```python
from build123d import *

# Parameters (mm, degrees)
SKETCH_1_R                   = 27.5
SKETCH_1_R_2                 = 17.5
EXTRUDE_1_DEPTH              = 4
SKETCH_2_R                   = 27.5
SKETCH_2_R_2                 = 18.5
EXTRUDE_2_DEPTH              = 5
EXTRUDE_3_DEPTH              = 9
SKETCH_7_R                   = 18.5
CUT_EXTRUDE_4_DEPTH          = 3
SKETCH_13_R                  = 9.5
CUT_EXTRUDE_9_DEPTH          = 7
SKETCH_14_R                  = 8.5
CUT_EXTRUDE_10_DEPTH         = 3
SKETCH_26_W                  = 65.286774434
SKETCH_26_H                  = 13.225755288
CUT_EXTRUDE_11_DEPTH         = 1111
SKETCH_28_R                  = 9.5
SKETCH_28_R_2                = 8.5
EXTRUDE_4_DEPTH              = 2
HOLE_WIZARD_M3_1_D           = 3.2
HOLE_WIZARD_M3_1_CBORE_D     = 6.5
HOLE_WIZARD_M3_1_CBORE_DEPTH = 3.4
PATTERN_CIRCULAR_1_COUNT     = 6
HOLE_WIZARD_M3_2_D           = 3.2
HOLE_WIZARD_M3_2_CBORE_D     = 6.5
HOLE_WIZARD_M3_2_CBORE_DEPTH = 3.4
PATTERN_CIRCULAR_2_COUNT     = 6


with BuildPart() as part:
    # 스케치1 → 보스-돌출1 (new body)
    with BuildSketch(Plane(origin=(0, 0, 0), x_dir=(1, 0, 0), z_dir=(0, 1, 0))):
        Circle(SKETCH_1_R)
        Circle(SKETCH_1_R_2, mode=Mode.SUBTRACT)
    extrude(amount=EXTRUDE_1_DEPTH)

    # 스케치2 → 보스-돌출2 (add)
    with BuildSketch(Plane(origin=(0, 4, 0), x_dir=(1, 0, 0), z_dir=(0, 1, 0))):
        Circle(SKETCH_2_R)
        Circle(SKETCH_2_R_2, mode=Mode.SUBTRACT)
    extrude(amount=EXTRUDE_2_DEPTH)

    # 스케치3 → 보스-돌출3 (add)
    with BuildSketch(Plane(origin=(0, 9, 0), x_dir=(1, 0, 0), z_dir=(0, 1, 0))):
        with BuildLine():
            Line((4.125, 27.188864908), (62.775, 18.290690938))
            ThreePointArc((62.775, 18.290690938), (78.5, 0), (62.775, -18.290690938))
            Line((62.775, -18.290690938), (4.125, -27.188864908))
            ThreePointArc((4.125, -27.188864908), (27.5, 0), (4.125, 27.188864908))
        make_face()
    extrude(amount=-EXTRUDE_3_DEPTH)

    # 스케치7 → 컷-돌출4 (cut)
    with BuildSketch(Plane(origin=(0, 4, 0), x_dir=(1, 0, 0), z_dir=(0, 1, 0))):
        Circle(SKETCH_7_R)
    extrude(amount=-CUT_EXTRUDE_4_DEPTH, mode=Mode.SUBTRACT)

    # 스케치13 → 컷-돌출9 (cut)
    with BuildSketch(Plane.XZ):
        with Locations((60, 0)):
            Circle(SKETCH_13_R)
    extrude(amount=-CUT_EXTRUDE_9_DEPTH, mode=Mode.SUBTRACT)

    # 스케치14 → 컷-돌출10 (cut, through all)
    with BuildSketch(Plane.XZ.offset(-7)):
        with Locations((60, 0)):
            Circle(SKETCH_14_R)
    extrude(amount=-CUT_EXTRUDE_10_DEPTH, mode=Mode.SUBTRACT)

    # 스케치26 → 컷-돌출11 (cut, symmetric)
    with BuildSketch(Plane(origin=(0, 0, 0), x_dir=(0, 0, -1), z_dir=(1, 0, 0))):
        with Locations((-1.179133759, 11.612877644)):
            Rectangle(SKETCH_26_W, SKETCH_26_H)
    extrude(amount=CUT_EXTRUDE_11_DEPTH, both=True, mode=Mode.SUBTRACT)

    # 스케치28 → 보스-돌출4 (add)
    with BuildSketch(Plane.XZ):
        with Locations((60, 0)):
            Circle(SKETCH_28_R)
        with Locations((60, 0)):
            Circle(SKETCH_28_R_2, mode=Mode.SUBTRACT)
    extrude(amount=-EXTRUDE_4_DEPTH)

    # M3 육각 소켓 머리 캡 나사용 카운터보어1 (through all)
    with Locations(Plane(origin=(0, 0, 0), x_dir=(-1, 0, 0), z_dir=(0, -1, 0))):
        with Locations((0, 22.5)):
            hole_wizard_m3_1 = CounterBoreHole(HOLE_WIZARD_M3_1_D / 2, HOLE_WIZARD_M3_1_CBORE_D / 2, HOLE_WIZARD_M3_1_CBORE_DEPTH)

    # 원형 패턴1: M3 육각 소켓 머리 캡 나사용 카운터보어1 ×6 about axis
    pattern_circular_1_axis = Axis((0, 0, 0), (0, 1, 0))
    for i in range(1, PATTERN_CIRCULAR_1_COUNT):
        add(hole_wizard_m3_1.rotate(pattern_circular_1_axis, i * 360 / PATTERN_CIRCULAR_1_COUNT), mode=Mode.SUBTRACT)

    # M3 육각 소켓 머리 캡 나사용 카운터보어2 (through all)
    with Locations(Plane(origin=(0, 0, 0), x_dir=(-1, 0, 0), z_dir=(0, -1, 0))):
        with Locations((-60, 13.5)):
            hole_wizard_m3_2 = CounterBoreHole(HOLE_WIZARD_M3_2_D / 2, HOLE_WIZARD_M3_2_CBORE_D / 2, HOLE_WIZARD_M3_2_CBORE_DEPTH)

    # 원형 패턴2: M3 육각 소켓 머리 캡 나사용 카운터보어2 ×6 about axis
    pattern_circular_2_axis = Axis((60, 0, 0), (0, 1, 0))
    for i in range(1, PATTERN_CIRCULAR_2_COUNT):
        add(hole_wizard_m3_2.rotate(pattern_circular_2_axis, i * 360 / PATTERN_CIRCULAR_2_COUNT), mode=Mode.SUBTRACT)


solid = part.part
```
Source: CAD feature listing. Evaluate the final solid. Frame: model axes, mm. A direction names the side the tool comes from. Round coordinates to 2 decimals unless told otherwise and drop trailing zeros. Loops run counter-clockwise (first coordinate to the right, second up) from the corner with the lowest first, then second, coordinate; pieces in that order, holes last.
(1) Contact query for flat-ended pins moving along their axis: pin 1 Ø5 at (x, z) = (-20, -11) entering from -Y; pin 2 Ø2 at (x, y) = (-10, 3) entering from -Z; pin 3 Ø2.5 at (x, z) = (60, 13.5) entering from -Y. Output: stop coordinate, or through.
From the geometry:
pin 1: stops at y = 3.4
pin 2: stops at z = -25.99
pin 3: passes through
(2) Material intervals for probe 1 along X at (y, z) = (3.8, -3); probe 2 along X at (y, z) = (2.05, -6.5); probe 3 along X at (y, z) = (0.45, -15), sorted ascending.
From the geometry:
probe 1: x = -27.34 to -18.26, 18.26 to 50.99, 69.01 to 78.26
probe 2: x = -26.72 to -17.32, 17.32 to 45.07, 51.55 to 53.07, 66.93 to 68.45, 74.93 to 77.32
probe 3: x = -23.05 to -9.01, 9.01 to 57.12, 62.88 to 70.83
(3) Section query D-D (x = 60). Output: boundary loops of the cut face in (y, z), and give its area (3 significant figures).
From the geometry:
outline: (0, -18.71) - (5, -18.71) - (5, -15.1) - (3.4, -15.1) - (3.4, -16.75) - (0, -16.75) - close; (0, -10.25) - (3.4, -10.25) - (3.4, -11.9) - (5, -11.9) - (5, -9.5) - (2, -9.5) - (2, -8.5) - (0, -8.5) - close; (0, 8.5) - (2, 8.5) - (2, 9.5) - (5, 9.5) - (5, 11.9) - (3.4, 11.9) - (3.4, 10.25) - (0, 10.25) - close; (0, 16.75) - (3.4, 16.75) - (3.4, 15.1) - (5, 15.1) - (5, 18.71) - (0, 18.71) - close
area: 41.7 mm2
(4) Section query C-C (z = 22.5). Output: boundary loops of the cut face in (x, y), and give its area (3 significant figures).
From the geometry:
outline: (-15.81, 0) - (-3.25, 0) - (-3.25, 3.4) - (-1.6, 3.4) - (-1.6, 5) - (-15.81, 5) - close; (1.6, 3.4) - (3.25, 3.4) - (3.25, 0) - (35.03, 0) - (35.03, 5) - (1.6, 5) - close
area: 227 mm2
(5) Section query A-A (x = 0). Output: boundary loops of the cut face in (y, z), and give its area (3 significant figures).
From the geometry:
outline: (0, -27.5) - (5, -27.5) - (5, -24.1) - (3.4, -24.1) - (3.4, -25.75) - (0, -25.75) - close; (0, -19.25) - (3.4, -19.25) - (3.4, -20.9) - (5, -20.9) - (5, -18.5) - (1, -18.5) - (1, -17.5) - (0, -17.5) - close; (0, 17.5) - (1, 17.5) - (1, 18.5) - (5, 18.5) - (5, 20.9) - (3.4, 20.9) - (3.4, 19.25) - (0, 19.25) - close; (0, 25.75) - (3.4, 25.75) - (3.4, 24.1) - (5, 24.1) - (5, 27.5) - (0, 27.5) - close
area: 37.6 mm2
(6) Access query for faces 5 (the cylindrical face through (-18.306, 4.211, -10.169)), 6 (the cylindrical face through (-4.01, 2.97, 18.06)), 7 (the flat face through (19, 3.4, 13)). Directions: +Z, -Z, +X, -X, +Y, -Y. A direction counts if a zero-diameter tool reaches every point of the face in a straight line with its end or side. Return the directions, or none.
From the geometry:
face 5: +Y, -Y
face 6: +Y
face 7: -Y
(7) Section query B-B (z = 0). Output: boundary loops of the cut face in (x, y).
From the geometry:
outline: (-27.5, 0) - (-17.5, 0) - (-17.5, 1) - (-18.5, 1) - (-18.5, 5) - (-27.5, 5) - close; (17.5, 0) - (51.5, 0) - (51.5, 2) - (50.5, 2) - (50.5, 5) - (18.5, 5) - (18.5, 1) - (17.5, 1) - close; (68.5, 0) - (78.5, 0) - (78.5, 5) - (69.5, 5) - (69.5, 2) - (68.5, 2) - close
(8) Pull-direction query (Z, two-part tool) for faces 1 (the cylindrical face through (78.496, 2.535, -0.368)), 2 (the cylindrical face through (73.29, 4.21, -6.68)), 3 (the flat face through (26, 5, 0)), 4 (the cylindrical face through (-0.208, 4.211, -24.086)); classes: +Z half, -Z half, draft (parallel to the pull), parting line (faces both ways), or undercut.
From the geometry:
face 1: parting line
face 2: undercut
face 3: draft
face 4: undercut
